For this review, take the finished solid that the model builds, in its own axes (mm). A direction names the side the tool comes from. Round coordinates to 2 decimals unless told otherwise and drop trailing zeros. Loops run counter-clockwise (first coordinate to the right, second up) from the corner with the lowest first, then second, coordinate; pieces in that order, holes last. Notation, with made-up numbers: M 19,-39.5 L 63,-39.5 A22 cw 63,-4.5 Z; hole C 49,70.25 d1. An arc over 180 degrees is marked long. Write item = value, one per line. Start each with the question number.
```python
from build123d import *

# Parameters (mm, degrees)
SKETCH2_R                = 8.5
CUT_EXTRUDE1_DEPTH       = 10
CIRPATTERN1_COUNT        = 4
CUT_EXTRUDE2_DEPTH       = 12
F_4_0_4_DIAMETER_HOLE1_D = 4


with BuildPart() as part:
    # Sketch1 → Revolve3 (revolve)
    with BuildSketch(Plane.XY):
        with BuildLine():
            Line((0, 81.005557052), (-10, 81.005557052))
            ThreePointArc((-10, 81.005557052), (-8.823173444, 75.522629002), (-5.5, 71.005557052))
            Line((-5.5, 71.005557052), (-5.5, 66.005557052))
            add(Edge.make_bspline(
                [(-5.5, 66.005557052), (-4.587686539, 56.99839644), (-5.5, 48.005557052)],
                knots=[0, 0, 0, 1, 1, 1], degree=2))
            Line((-5.5, 48.005557052), (-5.5, 43.005557052))
            Line((-5.5, 43.005557052), (0, 43.005557052))
            Line((0, 43.005557052), (0, 81.005557052))
        make_face()
    revolve(axis=Axis((0, 81.005557052, 0), (0, -1, 0)))

    # Sketch2 → Cut-Extrude1 (cut)
    with BuildSketch(Plane(origin=(0, 81.005557052, 0), x_dir=(1, 0, 0), z_dir=(0, 1, 0))):
        with Locations((0, 15.36427344)):
            Circle(SKETCH2_R)
    cut_extrude1 = extrude(amount=-CUT_EXTRUDE1_DEPTH, mode=Mode.SUBTRACT)

    # CirPattern1: Cut-Extrude1 ×4 about axis
    cirpattern1_axis = Axis((0, 0, 0), (0, 1, 0))
    for i in range(1, CIRPATTERN1_COUNT):
        add(cut_extrude1.rotate(cirpattern1_axis, i * 360 / CIRPATTERN1_COUNT), mode=Mode.SUBTRACT)

    # Sketch3 → Cut-Extrude2 (cut)
    with BuildSketch(Plane(origin=(0, 81.005557052, 0), x_dir=(1, 0, 0), z_dir=(0, 1, 0))):
        Polygon((-2.598076211, 4.5), (-5.196152423, 0), (-2.598076211, -4.5), (2.598076211, -4.5), (5.196152423, 0), (2.598076211, 4.5), align=None)
    extrude(amount=-CUT_EXTRUDE2_DEPTH, mode=Mode.SUBTRACT)

    # Ø4.0 (4) Diameter Hole1 (through all)
    with Locations(Plane(origin=(0, 69.005557052, 0), x_dir=(1, 0, 0), z_dir=(0, 1, 0))):
        with Locations((0, 0)):
            Hole(F_4_0_4_DIAMETER_HOLE1_D / 2)


solid = part.part
```
(1) Draft analysis for pull direction X (two halves, no side actions). For faces 1 (the flat face through (-3.88, 75.09, -2.28)), 2 (the cylindrical face through (6.865, 77.721, -0.077)), 3 (the flat face through (0.1, 43.006, 2.4)), state which applies: +X half, -X half, draft (parallel to the pull), parting line (faces both ways), or undercut.
(2) Tool access review of faces 4 (the cylindrical face through (1.19, 68.47, 5.37)), 5 (the cylindrical face through (0, 56, 2)), 6 (the flat face through (3.915, 75.09, -2.219)): name each direction out of +Z, -Z, +X, -X, +Y, -Y from which nothing blocks a thin tool from reaching the whole face with its end or side.
(3) Add section A-A on y = 68. Write out the cut boundary in (x, z), and give its area (3 significant figures).
(4) For pin 1 Ø1.6 at (x, y) = (-1, 76) entering from +Z; pin 2 Ø4 at (x, y) = (0.5, 76) entering from -Z; pin 3 Ø3 at (y, z) = (70.5, -5.5) entering from +X, all flat-tipped, find the tip position at first contact; note any pin that passes through.
(5) Wall thickness on L1, parallel to Y at x = 2.25, z = 2; L2, parallel to Z at x = 0, y = 54; L3, parallel to Z at x = 0.5, y = 72: over which ranges is each line inside the solid? List them lowest first.
Answer sheet:
q1.face_1 = undercut
q1.face_2 = +X half
q1.face_3 = draft
q2.face_4 = -Y
q2.face_5 = +Y, -Y
q2.face_6 = +Y
q3.outline = C 0,0 d11; hole C 0,0 d4
q3.area = 82.5 mm²
q4.pin_1 = 7.06
q4.pin_2 = -7.24
q4.pin_3 = 4.2
q5.L1 = 43.01 to 69.01
q5.L2 = -5.09 to -2, 2 to 5.09
q5.L3 = -6.49 to -4.5, 4.5 to 6.49
